Read the model definition and answer for the solid it produces. Units are mm, in the model's axes. A direction names the side the tool comes from. Coordinates: 2 decimals unless noted, no trailing zeros. Loops run counter-clockwise (first coordinate to the right, second up) from the corner with the lowest first, then second, coordinate; pieces in that order, holes last. Notation, with made-up numbers: (30.25, -5.5) -> (73.25, -5.5) arc R14 cw to (73.25, 1.5) -> close; hole circle Ø4 at (4.5, 9). An arc over 180 degrees is marked (long way). Answer in a Markdown table with one row per item.
```python
from build123d import *

# Parameters (mm, degrees)
SKETCH1_R           = 1.75
BOSS_EXTRUDE1_DEPTH = 4
BOSS_EXTRUDE2_START = -4
SKETCH2_R           = 1.6
SKETCH2_R_2         = 2.35
BOSS_EXTRUDE2_DEPTH = 4
FILLET1_R           = 2


with BuildPart() as part:
    # Sketch1 → Boss-Extrude1 (new body)
    with BuildSketch(Plane.XY):
        with BuildLine():
            Line((6.458174517, 10.22648556), (7.730280052, 9.302246788))
            ThreePointArc((7.730280052, 9.302246788), (8.293531937, 9.074228241), (8.884801529, 9.214390334))
            ThreePointArc((8.884801529, 9.214390334), (9.700788202, 9.679292345), (10.537793023, 10.105192636))
            ThreePointArc((10.537793023, 10.105192636), (11.811648118, 8.581664683), (12.866966432, 6.899360466))
            ThreePointArc((12.866966432, 6.899360466), (12.203262471, 6.234932004), (11.508960635, 5.602545185))
            ThreePointArc((11.508960635, 5.602545185), (11.192946211, 5.083526854), (11.235750332, 4.477380873))
            Line((11.235750332, 4.477380873), (11.721651409, 2.981931127))
            ThreePointArc((11.721651409, 2.981931127), (12.043305816, 2.466389096), (12.604038176, 2.232243064))
            ThreePointArc((12.604038176, 2.232243064), (13.537447807, 2.12873176), (14.464936842, 1.981313243))
            ThreePointArc((14.464936842, 1.981313243), (14.6, 0), (14.464936842, -1.981313243))
            ThreePointArc((14.464936842, -1.981313243), (13.537447807, -2.12873176), (12.604038176, -2.232243064))
            ThreePointArc((12.604038176, -2.232243064), (12.043305816, -2.466389096), (11.721651409, -2.981931127))
            Line((11.721651409, -2.981931127), (11.235750332, -4.477380873))
            ThreePointArc((11.235750332, -4.477380873), (11.192946211, -5.083526854), (11.508960635, -5.602545185))
            ThreePointArc((11.508960635, -5.602545185), (12.203262471, -6.234932004), (12.866966432, -6.899360466))
            ThreePointArc((12.866966432, -6.899360466), (11.811648118, -8.581664683), (10.537793023, -10.105192636))
            ThreePointArc((10.537793023, -10.105192636), (9.700788202, -9.679292345), (8.884801529, -9.214390334))
            ThreePointArc((8.884801529, -9.214390334), (8.293531937, -9.074228241), (7.730280052, -9.302246788))
            Line((7.730280052, -9.302246788), (6.458174517, -10.22648556))
            ThreePointArc((6.458174517, -10.22648556), (6.067261587, -10.691708329), (6.017851306, -11.297351596))
            ThreePointArc((6.017851306, -11.297351596), (6.207845644, -12.21706366), (6.354252177, -13.144712978))
            ThreePointArc((6.354252177, -13.144712978), (4.511648118, -13.885425138), (2.585570436, -14.369231904))
            ThreePointArc((2.585570436, -14.369231904), (2.158757221, -13.532692241), (1.771872682, -12.676953681))
            ThreePointArc((1.771872682, -12.676953681), (1.375910744, -12.216020619), (0.786204458, -12.069420349))
            Line((0.786204458, -12.069420349), (-0.786204458, -12.069420349))
            ThreePointArc((-0.786204458, -12.069420349), (-1.375910744, -12.216020619), (-1.771872682, -12.676953681))
            ThreePointArc((-1.771872682, -12.676953681), (-2.158757221, -13.532692241), (-2.585570436, -14.369231904))
            ThreePointArc((-2.585570436, -14.369231904), (-4.511648118, -13.885425138), (-6.354252177, -13.144712978))
            ThreePointArc((-6.354252177, -13.144712978), (-6.207845644, -12.21706366), (-6.017851306, -11.297351596))
            ThreePointArc((-6.017851306, -11.297351596), (-6.067261587, -10.691708329), (-6.458174517, -10.22648556))
            Line((-6.458174517, -10.22648556), (-7.730280052, -9.302246788))
            ThreePointArc((-7.730280052, -9.302246788), (-8.293531937, -9.074228241), (-8.884801529, -9.214390334))
            ThreePointArc((-8.884801529, -9.214390334), (-9.700788202, -9.679292345), (-10.537793023, -10.105192636))
            ThreePointArc((-10.537793023, -10.105192636), (-11.811648118, -8.581664683), (-12.866966432, -6.899360466))
            ThreePointArc((-12.866966432, -6.899360466), (-12.203262471, -6.234932004), (-11.508960635, -5.602545185))
            ThreePointArc((-11.508960635, -5.602545185), (-11.192946211, -5.083526854), (-11.235750332, -4.477380873))
            Line((-11.235750332, -4.477380873), (-11.721651409, -2.981931127))
            ThreePointArc((-11.721651409, -2.981931127), (-12.043305816, -2.466389096), (-12.604038176, -2.232243064))
            ThreePointArc((-12.604038176, -2.232243064), (-13.537447807, -2.12873176), (-14.464936842, -1.981313243))
            ThreePointArc((-14.464936842, -1.981313243), (-14.6, 0), (-14.464936842, 1.981313243))
            ThreePointArc((-14.464936842, 1.981313243), (-13.537447807, 2.12873176), (-12.604038176, 2.232243064))
            ThreePointArc((-12.604038176, 2.232243064), (-12.043305816, 2.466389096), (-11.721651409, 2.981931127))
            Line((-11.721651409, 2.981931127), (-11.235750332, 4.477380873))
            ThreePointArc((-11.235750332, 4.477380873), (-11.192946211, 5.083526854), (-11.508960635, 5.602545185))
            ThreePointArc((-11.508960635, 5.602545185), (-12.203262471, 6.234932004), (-12.866966432, 6.899360466))
            ThreePointArc((-12.866966432, 6.899360466), (-11.811648118, 8.581664683), (-10.537793023, 10.105192636))
            ThreePointArc((-10.537793023, 10.105192636), (-9.700788202, 9.679292345), (-8.884801529, 9.214390334))
            ThreePointArc((-8.884801529, 9.214390334), (-8.293531937, 9.074228241), (-7.730280052, 9.302246788))
            Line((-7.730280052, 9.302246788), (-6.458174517, 10.22648556))
            ThreePointArc((-6.458174517, 10.22648556), (-6.067261587, 10.691708329), (-6.017851306, 11.297351596))
            ThreePointArc((-6.017851306, 11.297351596), (-6.207845644, 12.21706366), (-6.354252177, 13.144712978))
            ThreePointArc((-6.354252177, 13.144712978), (-4.511648118, 13.885425138), (-2.585570436, 14.369231904))
            ThreePointArc((-2.585570436, 14.369231904), (-2.158757221, 13.532692241), (-1.771872682, 12.676953681))
            ThreePointArc((-1.771872682, 12.676953681), (-1.375910744, 12.216020619), (-0.786204458, 12.069420349))
            Line((-0.786204458, 12.069420349), (0.786204458, 12.069420349))
            ThreePointArc((0.786204458, 12.069420349), (1.375910744, 12.216020619), (1.771872682, 12.676953681))
            ThreePointArc((1.771872682, 12.676953681), (2.158757221, 13.532692241), (2.585570436, 14.369231904))
            ThreePointArc((2.585570436, 14.369231904), (4.511648118, 13.885425138), (6.354252177, 13.144712978))
            ThreePointArc((6.354252177, 13.144712978), (6.207845644, 12.21706366), (6.017851306, 11.297351596))
            ThreePointArc((6.017851306, 11.297351596), (6.067261587, 10.691708329), (6.458174517, 10.22648556))
        make_face()
        Circle(SKETCH1_R, mode=Mode.SUBTRACT)
    extrude(amount=BOSS_EXTRUDE1_DEPTH)

    # Sketch2 → Boss-Extrude2 (add)
    with BuildSketch(Plane(origin=(0, 0, 0), x_dir=(-1, 0, 0), z_dir=(0, 0, -1)).offset(BOSS_EXTRUDE2_START)):
        with BuildLine():
            Line((7.965480191, 7.845452525), (46.007740843, 20.2061323))
            ThreePointArc((46.007740843, 20.2061323), (52.308108396, 16.995934691), (49.097910787, 10.695567137))
            Line((49.097910787, 10.695567137), (11.055650135, -1.665112638))
            Line((11.055650135, -1.665112638), (7.965480191, 7.845452525))
        make_face()
        with Locations((47.552825815, 15.450849719)):
            Circle(SKETCH2_R, mode=Mode.SUBTRACT)
        with Locations((39.963394815, 12.984894104)):
            Circle(SKETCH2_R_2, mode=Mode.SUBTRACT)
        with Locations((32.373963815, 10.518938489)):
            Circle(SKETCH2_R, mode=Mode.SUBTRACT)
        with Locations((24.784532815, 8.052982873)):
            Circle(SKETCH2_R_2, mode=Mode.SUBTRACT)
        with Locations((17.195101815, 5.587027258)):
            Circle(SKETCH2_R, mode=Mode.SUBTRACT)
    extrude(amount=BOSS_EXTRUDE2_DEPTH)

    # Fillet1
    # the kernel refuses this fillet: 2 mm, written as the material it takes off along each edge
    with BuildSketch(Plane(origin=(-14.464936842, -1.981313243, -4.187001337), x_dir=(-0.08564855994772169, 0.9963254107864967, 0), z_dir=(0, 0, 1))) as fillet1_piece_1:
        with BuildLine():
            CenterArc((1.593192122, -1.99621856), FILLET1_R, 93.523868458, 76.001739978)
            Line((-0.373480398, -1.63262648), (-0.412813848, -1.625354638))
            ThreePointArc((-0.412813848, -1.625354638), (-0.242909966, -0.803463818), (-0.038582997, 0.010552361))
            Line((-0.038582997, 0.010552361), (-0.00201406, 0.039949262))
            ThreePointArc((-0.00201406, 0.039949262), (0.73513172, 0.058519233), (1.467804867, 0.039924371))
            Line((1.467804867, 0.039924371), (1.470263441, 0))
        make_face()
    extrude(amount=12.374002673, mode=Mode.SUBTRACT)
    with BuildSketch(Plane(origin=(-10.537793023, 10.105192636, -4.187001337), x_dir=(0.8827178463652419, -0.4699033982727826, 0), z_dir=(0, 0, 1))) as fillet1_piece_2:
        with BuildLine():
            CenterArc((1.590668977, -1.998229687), FILLET1_R, 87.589097028, 76.001739978)
            Line((-0.327868641, -1.433239945), (-0.366239393, -1.42194015))
            ThreePointArc((-0.366239393, -1.42194015), (-0.220979949, -0.703570188), (-0.038494143, 0.010872025))
            Line((-0.038494143, 0.010872025), (-0.001682631, 0.039964594))
            ThreePointArc((-0.001682631, 0.039964594), (0.837400267, 0.057620746), (1.676483166, 0.039964594))
            Line((1.676483166, 0.039964594), (1.674800535, 0))
        make_face()
    extrude(amount=12.374002673, mode=Mode.SUBTRACT)
    with BuildSketch(Plane(origin=(-6.354252177, 13.144712978, -4.315988382), x_dir=(0.9244796007365503, 0.3812315147282405, 0), z_dir=(0, 0, 1)), Plane(origin=(2.585570436, 14.369231904, -4.315988382), x_dir=(0.9720019700152155, -0.23497270115172955, 0), z_dir=(0, 0, 1)), Plane(origin=(10.537793023, 10.105192636, -4.315988382), x_dir=(0.6482526238799229, -0.7614253316201104, 0), z_dir=(0, 0, 1)), Plane(origin=(14.464936842, 1.981313243, -4.315988382), x_dir=(0.07689280871880408, -0.9970393653047674, 0), z_dir=(0, 0, 1)), Plane(origin=(12.866966432, -6.899360466, -4.315988382), x_dir=(-0.5238374458824551, -0.8518182495646274, 0), z_dir=(0, 0, 1)), Plane(origin=(6.354252177, -13.144712978, -4.315988382), x_dir=(-0.9244796007365504, -0.3812315147282399, 0), z_dir=(0, 0, 1)), Plane(origin=(-2.585570436, -14.369231904, -4.315988382), x_dir=(-0.9720019700152157, 0.23497270115172855, 0), z_dir=(0, 0, 1)), Plane(origin=(-10.537793023, -10.105192636, -4.315988382), x_dir=(-0.6482526238799226, 0.7614253316201107, 0), z_dir=(0, 0, 1))) as fillet1_piece_3:
        with BuildLine():
            CenterArc((1.608149096, -1.996501396), FILLET1_R, 86.610517624, 83.465059025)
            Line((-0.361922802, -1.651803385), (-0.40132424, -1.644909425))
            ThreePointArc((-0.40132424, -1.644909425), (-0.237581401, -0.813495816), (-0.038674208, 0.010213013))
            Line((-0.038674208, 0.010213013), (-0.002364925, 0.039930028))
            ThreePointArc((-0.002364925, 0.039930028), (0.863197676, 0.065539812), (1.728760278, 0.039930028))
            Line((1.728760278, 0.039930028), (1.726395353, 0))
        make_face()
    extrude(amount=12.631976765, mode=Mode.SUBTRACT)
    with BuildSketch(Plane(origin=(-2.585570436, 14.369231904, -4.315988382), x_dir=(0.43756555631998817, -0.8991865123111997, 0), z_dir=(0, 0, 1)), Plane(origin=(6.354252177, 13.144712978, -4.315988382), x_dir=(-0.1745305997808264, -0.9846517504885395, 0), z_dir=(0, 0, 1)), Plane(origin=(12.866966432, 6.899360466, -4.315988382), x_dir=(-0.719961998842273, -0.6940134870613388, 0), z_dir=(0, 0, 1)), Plane(origin=(14.464936842, -1.981313243, -4.315988382), x_dir=(-0.9903923849542835, -0.13828566022753844, 0), z_dir=(0, 0, 1)), Plane(origin=(10.537793023, -10.105192636, -4.315988382), x_dir=(-0.8825265422128264, 0.47026258865645726, 0), z_dir=(0, 0, 1)), Plane(origin=(2.585570436, -14.369231904, -4.315988382), x_dir=(-0.4375655563199897, 0.899186512311199, 0), z_dir=(0, 0, 1)), Plane(origin=(-6.354252177, -13.144712978, -4.315988382), x_dir=(0.17453059978082774, 0.9846517504885393, 0), z_dir=(0, 0, 1)), Plane(origin=(-12.866966432, -6.899360466, -4.315988382), x_dir=(0.7199619988422736, 0.694013487061338, 0), z_dir=(0, 0, 1))) as fillet1_piece_4:
        with BuildLine():
            CenterArc((1.606043881, -1.998195283), FILLET1_R, 87.565780038, 83.465059025)
            Line((-0.369500914, -1.686389632), (-0.40901181, -1.680153518))
            ThreePointArc((-0.40901181, -1.680153518), (-0.248771516, -0.82916731), (-0.038498565, 0.010856359))
            Line((-0.038498565, 0.010856359), (-0.001698895, 0.039963906))
            ThreePointArc((-0.001698895, 0.039963906), (0.845494314, 0.05796318), (1.692687522, 0.039963906))
            Line((1.692687522, 0.039963906), (1.690988628, 0))
        make_face()
    extrude(amount=12.631976765, mode=Mode.SUBTRACT)


solid = part.part
```
1. The mould has two halves that part along X. Classify faces 5 (the cylindrical face through (-14.004, -1.659, 1.972)), 6 (the flat face through (-28.51, 14.52, 2.03)), 7 (the cylindrical face through (5.84, -12.91, 1.97)): pulls with the +X half, pulls with the -X half, needs draft (parallel to the pull), parting line crosses it, or undercut.
A:
| item | result |
|---|---|
| face 5 | pulls with the -X half |
| face 6 | undercut |
| face 7 | pulls with the +X half |
2. A cutting plane is placed at B-B on x = -39. Give the vertices of the cut face in (y, z), and give its area (3 significant figures).
A:
| item | result |
|---|---|
| outline | (7.41, 0) -> (10.84, 0) -> (10.84, 4) -> (7.41, 4) -> close; (15.13, 0) -> (17.93, 0) -> (17.93, 4) -> (15.13, 4) -> close |
| area | 24.9 mm2 |
3. A cutting plane is placed at C-C on z = 2.9. Count the separate pieces of the cut face and the enclosed holes in it, and give its area (3 significant figures).
A:
| item | result |
|---|---|
| separate pieces | 1 |
| enclosed holes | 6 |
| area | 898 mm2 |
4. A tool of negligible diameter and unlimited length cuts with its end or side. For faces 1 (the flat face through (-11.475, -3.74, 1.972)), 2 (the flat face through (7.1, -9.76, 1.97)), 3 (the flat face through (7.085, 9.771, 1.972)), 4 (the cylindrical face through (12.308, 6.968, 1.972)), from which of +Z, -Z, +X, -X, +Y, -Y can it reach the whole face along a straight path? Write none if from no direction.
A:
| item | result |
|---|---|
| face 1 | +Z, -Z, -X |
| face 2 | +Z, -Z, -Y |
| face 3 | +Z, -Z, +Y |
| face 4 | +Z, -Z, +X |
5. Given pin 1 Ø1 at (y, z) = (-9, 1) entering from +X; pin 2 Ø1.7 at (x, z) = (-0.5, 1.5) entering from +Y; pin 3 Ø5.5 at (x, y) = (-24.78, 8.05) entering from -Z; pin 4 Ø0.5 at (x, z) = (0, 2) entering from -Y, each flat-ended and moving along its own axis, determine where each tip first touches the part or whether it passes through.
A:
| item | result |
|---|---|
| pin 1 | stops at x = 11.87 |
| pin 2 | stops at y = 12.2 |
| pin 3 | stops at z = 0 |
| pin 4 | stops at y = -12.07 |
6. A cutting plane is placed at D-D on y = -7. Give the vertices of the cut face in (x, z).
A:
| item | result |
|---|---|
| outline | (-12.31, 0) -> (12.31, 0) -> (12.31, 4) -> (-12.31, 4) -> close |
7. A cutting plane is placed at A-A on x = 0. Give the vertices of the cut face in (y, z).
A:
| item | result |
|---|---|
| outline | (-12.07, 0) -> (-1.75, 0) -> (-1.75, 4) -> (-12.07, 4) -> close; (1.75, 0) -> (12.07, 0) -> (12.07, 4) -> (1.75, 4) -> close |
8. Find the intervals of material crossed by probe 1 along Y at (x, z) = (0, 2.6); probe 2 along Y at (x, z) = (-40, 1.5); probe 3 along X at (y, z) = (-9, 3.65), in increasing order.
A:
| item | result |
|---|---|
| probe 1 | y = -12.07 to -1.75, 1.75 to 12.07 |
| probe 2 | y = 7.74 to 10.64, 15.33 to 18.25 |
| probe 3 | x = -11.47 to 11.47 |
